from build123d import *

# Parameters (mm, degrees)
BOSS_EXTRUDE1_DEPTH      = 30.3
CUT_EXTRUDE1_DEPTH       = 181.717957049
CUT_EXTRUDE7_DEPTH       = 27.29
CUT_EXTRUDE10_DEPTH      = 96
CUT_EXTRUDE11_DEPTH      = 48
SKETCH9_W                = 2
SKETCH9_H                = 7.4
BOSS_EXTRUDE2_DEPTH      = 1.5
FILLET8_R                = 1
CUT_EXTRUDE15_DEPTH      = 2.6
CUT_EXTRUDE15_DEPTH_BACK = 2.6
SKETCH10_W               = 29
SKETCH10_H               = 15.5
SKETCH11_W               = 3.45
SKETCH11_H               = 8
BOSS_EXTRUDE3_DEPTH      = 1.3
FILLET9_R                = 7
CUT_EXTRUDE18_DEPTH      = 2.5
CUT_EXTRUDE23_START      = -2.5
CUT_EXTRUDE23_DEPTH      = 2.5
SKETCH18_W               = 4.5
SKETCH18_H               = 15
SKETCH18_W_2             = 3.45
SKETCH18_H_2             = 8
CUT_EXTRUDE24_DEPTH      = 1


# Read off the part's stored shape, not the designer's step: Cut-Extrude23
# Some blends are built 0.0001 mm under size
with BuildPart() as part:
    # Sketch1 → Boss-Extrude1 (new body)
    with BuildSketch(Plane.XY):
        Polygon((34.45, 2), (35.7, 0), (53.3, 0), (53.3, 48), (45, 74), (45, 170), (0, 170), (0, 2), align=None)
    extrude(amount=BOSS_EXTRUDE1_DEPTH)

    # Sketch2 → Cut-Extrude1 (cut, through all)
    with BuildSketch(Plane(origin=(0, 170, 0), x_dir=(1, 0, 0), z_dir=(0, 1, 0))):
        with BuildLine():
            Line((0, -30.3), (9.25, -30.3))
            ThreePointArc((9.25, -30.3), (2.495291793, -24.025316905), (0, -15.150000022))
            Line((0, -15.150000022), (0, -30.3))
        make_face()
        with BuildLine():
            ThreePointArc((0, -15.150000022), (2.495291781, -6.274683113), (9.25, 0))
            Line((9.25, 0), (0, 0))
            Line((0, 0), (0, -15.150000022))
        make_face()
    extrude(amount=-CUT_EXTRUDE1_DEPTH, mode=Mode.SUBTRACT)

    # Sketch7 → Cut-Extrude7 (cut)
    with BuildSketch(Plane(origin=(-8.97657775, 28.11940018, 0), x_dir=(0, 0, -1), z_dir=(0.30411092373144827, -0.9526366285563479, 0))):
        with BuildLine():
            Line((-15.15, 65.372856641), (-30.3, 65.372856641))
            Line((-30.3, 65.372856641), (-30.3, 56.120928382))
            ThreePointArc((-30.3, 56.120928382), (-24.02581935, 62.876979624), (-15.15, 65.372856641))
        make_face()
        with BuildLine():
            Line((0, 65.372856641), (-15.15, 65.372856641))
            ThreePointArc((-15.15, 65.372856641), (-6.27418065, 62.876979624), (0, 56.120928382))
            Line((0, 56.120928382), (0, 65.372856641))
        make_face()
    extrude(amount=-CUT_EXTRUDE7_DEPTH, mode=Mode.SUBTRACT)

    # Sketch6 → Cut-Extrude10 (cut)
    with BuildSketch(Plane(origin=(0, 170, 0), x_dir=(1, 0, 0), z_dir=(0, 1, 0))):
        with BuildLine():
            Line((45, -15.15), (45, 0))
            Line((45, 0), (35.74807174, 0))
            ThreePointArc((35.74807174, 0), (42.504122982, -6.27418065), (45, -15.15))
        make_face()
        with BuildLine():
            Line((45, -30.3), (45, -15.15))
            ThreePointArc((45, -15.15), (42.504122982, -24.02581935), (35.74807174, -30.3))
            Line((35.74807174, -30.3), (45, -30.3))
        make_face()
    extrude(amount=-CUT_EXTRUDE10_DEPTH, mode=Mode.SUBTRACT)

    # Sketch4 → Cut-Extrude11 (cut)
    with BuildSketch(Plane.XZ):
        with BuildLine():
            Line((53.3, 15.15), (53.3, 30.3))
            Line((53.3, 30.3), (44.04807174, 30.3))
            ThreePointArc((44.04807174, 30.3), (50.804122982, 24.02581935), (53.3, 15.15))
        make_face()
        with BuildLine():
            Line((53.3, 0), (53.3, 15.15))
            ThreePointArc((53.3, 15.15), (50.804122982, 6.27418065), (44.04807174, 0))
            Line((44.04807174, 0), (53.3, 0))
        make_face()
    extrude(amount=-CUT_EXTRUDE11_DEPTH, mode=Mode.SUBTRACT)

    # Sketch9 → Boss-Extrude2 (add)
    with BuildSketch(Plane.XZ.offset(-2)):
        with Locations((3, 15.15)):
            Rectangle(SKETCH9_W, SKETCH9_H)
    extrude(amount=BOSS_EXTRUDE2_DEPTH)

    # Fillet8
    fillet8_edges = [part.edges().sort_by_distance(p)[0] for p in [
        (4, 1.25, 11.45),
        (2, 1.25, 11.45),
        (4, 1.25, 18.85),
        (2, 1.25, 18.85),
    ]]
    fillet(fillet8_edges, radius=FILLET8_R - 0.0001)  # a hair under: the kernel refuses the full size

    # Sketch10 → Cut-Extrude15 (cut, two sides: drawn at the far end of the back side and taken through both)
    with BuildSketch(Plane.XZ.offset(-2).offset(-CUT_EXTRUDE15_DEPTH_BACK)):
        with Locations((21, 15.15)):
            Rectangle(SKETCH10_W, SKETCH10_H)
    extrude(amount=CUT_EXTRUDE15_DEPTH + CUT_EXTRUDE15_DEPTH_BACK, mode=Mode.SUBTRACT)

    # Sketch11 → Boss-Extrude3 (add)
    with BuildSketch(Plane.XZ):
        with Locations((43.575, 15.15)):
            Rectangle(SKETCH11_W, SKETCH11_H)
    extrude(amount=BOSS_EXTRUDE3_DEPTH)

    # Fillet9
    # the kernel refuses this fillet: 7 mm, written as the material it takes off along each edge
    with BuildSketch(Plane(origin=(55.458124827, -1.3, 11.15), x_dir=(0, 1, 0), z_dir=(-1, 0, 0)), Plane(origin=(31.691875173, -1.3, 19.15), x_dir=(0, 1, 0), z_dir=(1, 0, 0))) as fillet9_piece_1:
        with BuildLine():
            CenterArc((7, -4.063249931), FILLET9_R, 144.516796045, 35.483203955)
            Line((0, -4.063249931), (-0.14, -4.063249931))
            Line((-0.14, -4.063249931), (-0.14, 0))
            Line((-0.14, 0), (0, 0.14))
            ThreePointArc((0, 0.14), (0.65, 0.14), (1.186, 0.081264999))
            Line((1.186, 0.081264999), (1.3, 0))
        make_face()
    extrude(amount=23.766249654, mode=Mode.SUBTRACT)

    # Sketch13 → Cut-Extrude18 (cut)
    with BuildSketch(Plane(origin=(0, 74, 0), x_dir=(1, 0, 0), z_dir=(0, 1, 0))):
        with BuildLine():
            Line((35.74807174, -30.3), (45, -30.3))
            Line((45, -30.3), (45, -15.15))
            ThreePointArc((45, -15.15), (42.504122982, -24.02581935), (35.74807174, -30.3))
        make_face()
    extrude(amount=-CUT_EXTRUDE18_DEPTH, mode=Mode.SUBTRACT)

    # Cut-Extrude23 outline → Cut-Extrude23 (cut)
    with BuildSketch(Plane(origin=(0, 74, 0), x_dir=(1, 0, 0), z_dir=(0, 1, 0)).offset(CUT_EXTRUDE23_START)):
        with BuildLine():
            ThreePointArc((44.999624541, -15.036915931), (44.999829684, -15.061319249), (45, -15.085722835))
            Line((45, -15.085722835), (45, 0))
            Line((45, 0), (35.74807174, 0))
            ThreePointArc((35.74807174, 0), (42.474573722, -6.225973939), (44.999624541, -15.036915931))
        make_face()
    extrude(amount=CUT_EXTRUDE23_DEPTH, mode=Mode.SUBTRACT)

    # Sketch18 → Cut-Extrude24 (cut)
    with BuildSketch(Plane.XZ):
        with Locations((43.575, 15.15)):
            Rectangle(SKETCH18_W, SKETCH18_H)
        with Locations((43.575, 15.15)):
            Rectangle(SKETCH18_W_2, SKETCH18_H_2, mode=Mode.SUBTRACT)
    extrude(amount=-CUT_EXTRUDE24_DEPTH, mode=Mode.SUBTRACT)


solid = part.part
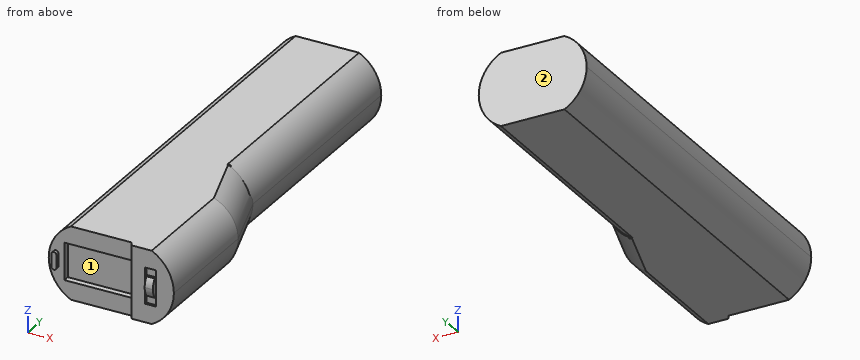
Verification items for the finished model (mm, model axes). Face numbers are marked on the shaded views. Give positions to 0.01 mm unless a question says otherwise; leave off trailing zeros. Write each loop counter-clockwise with the first axis right and the second up, starting at its lowest first coordinate (ties: lowest second). Pieces come first, ordered by that corner, then holes. Notation, with made-up numbers: (-24.75, -30.5) - (-4.75, -30.5) arc R11 cw to (-4.75, -19.5) - close; hole circle Ø9 at (-25.75, 57.5). An arc over 180 degrees is marked (long way). Answer as CSV lines item,"result". Start each with the question number.
1. Sectioned sample at C-C (y = 139.5). Record the boundary of the cut face in (x, z).
2. Draft check along X on the marked faces 1 and 2. Enter one of: pulls with the +X half, pulls with the -X half, needs draft (parallel to the pull), parting line crosses it, or undercut.
3. Thickness scan on line 1 (Y direction, x = 34.5, z = 15); line 2 (Y direction, x = 36, z = 28.5); line 3 (X direction, y = 154.5, z = 19.5). Record the ranges inside material, lowest first.
4. Depth check by flat-ended pin: pin 1 (0.7 mm diameter, centred on y = 0.5, z = 15, fed in from -X); pin 2 (2 mm diameter, centred on y = 73, z = 26, fed in from -X); pin 3 (1.6 mm diameter, centred on x = 2.5, z = 15.5, fed in from -Y). Enter the tip coordinate at first touch or a pass-through.
5. Sectioned sample at A-A (x = 32). Record the boundary of the cut face in (y, z).
Derived:
1,outline,"(9.25, 0) - (35.75, 0) arc R17.03 ccw to (35.75, 30.3) - (9.25, 30.3) arc R17.03 ccw to start"
2,face 1,"undercut"
2,face 2,"needs draft"
3,line 1,"4.6 to 170"
3,line 2,"0 to 170"
3,line 3,"0.56 to 44.44"
4,pin 1,"x = 2"
4,pin 2,"x = 3.14"
4,pin 3,"y = 0.5"
5,outline,"(2, 0) - (170, 0) - (170, 30.3) - (2, 30.3) - (2, 22.9) - (4.6, 22.9) - (4.6, 7.4) - (2, 7.4) - close"
